```python
from build123d import *

# Parameters (mm, degrees)
F1_DEPTH  = 1066.8
F3_W      = 101.6
F3_H      = 50.8
F4_DEPTH  = 152.4
F5_W      = 101.6
F5_H      = 50.8
F6_DEPTH  = 177.801
F8_DEPTH  = 177.801
F10_W     = 101.6
F10_H     = 101.6
F11_DEPTH = 177.801


with BuildPart() as f1:
    # F0 (on Top) → F1 (new body)
    with BuildSketch(Plane.XY):
        Polygon((76.2, 0), (0, 0), (0, -152.4), (558.8, -152.4), (558.8, 0), (482.6, 0), (482.6, 25.4), (330.2, 25.4), (330.2, 0), (228.6, 0), (228.6, 25.4), (76.2, 25.4), align=None)
    extrude(amount=F1_DEPTH)

    # F3 (on offset) → F4 (join)
    with BuildSketch(Plane.XZ.offset(152.4)):
        with Locations((279.4, 1092.2)):
            Rectangle(F3_W, F3_H)
    extrude(amount=-F4_DEPTH)

    # F5 (on offset) → F6 (cut, through all)
    with BuildSketch(Plane.XZ.offset(152.4)):
        with Locations((279.4, 25.4)):
            Rectangle(F5_W, F5_H)
    extrude(amount=-F6_DEPTH, mode=Mode.SUBTRACT)

    # F7 (on offset) → F8 (cut, through all)
    with BuildSketch(Plane.XZ.offset(152.4)):
        Polygon((586.1058764434, 586.1058764434), (0, 0), (586.1058764434, 0), align=None)
    extrude(amount=-F8_DEPTH, mode=Mode.SUBTRACT)

    # F9: F1 across face


with BuildPart() as f1_1:
    add(f1.part)
    add(f1.part.mirror(Plane(origin=(279.4, -68.7916666667, 279.4), x_dir=(0, 1, 0), z_dir=(0.7071067812, 0, -0.7071067812))))

    # F10 (on offset) → F11 (cut, through all)
    with BuildSketch(Plane.XZ.offset(152.4)):
        with Locations((279.4, 1066.8)):
            Rectangle(F10_W, F10_H)
    extrude(amount=-F11_DEPTH, mode=Mode.SUBTRACT)


solid = f1_1.part
```
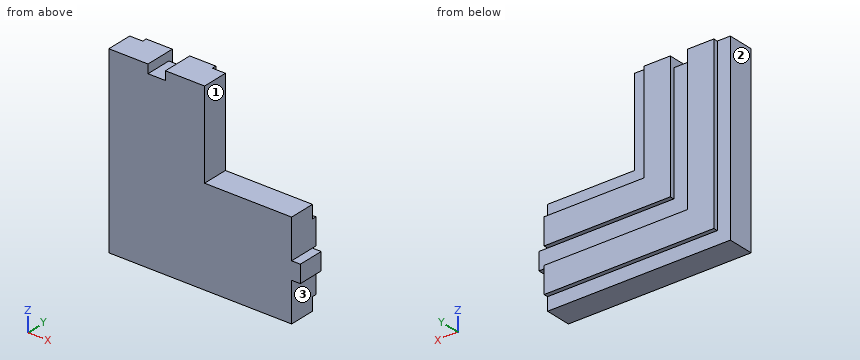
Input: part model. Units: mm. Frame: model coordinates. Face numbers are marked on the shaded views. A direction names the side the tool comes from. Round coordinates to 2 decimals unless told otherwise and drop trailing zeros. Loops run counter-clockwise (first coordinate to the right, second up) from the corner with the lowest first, then second, coordinate; pieces in that order, holes last. Notation, with made-up numbers: (-2.5, 21) -> (38.5, 21) arc R10 cw to (38.5, 39) -> close; hole circle Ø10 at (77.5, 33). An arc over 180 degrees is marked (long way). One line per item, written item: value.
(1) Material intervals for line 1 (Z direction, x = 677, y = 9); line 2 (X direction, y = -142.5, z = 534); line 3 (Z direction, x = 957, y = -5), sorted ascending. Write a range as [from, to].
Geometry check:
line 1: [76.2, 228.6], [330.2, 482.6]
line 2: [0, 1066.8]
line 3: [0, 558.8]
(2) Pin query (flat end, axial travel): pin 1 (7.5 mm diameter, centred on y = 6.5, z = 644, fed in from -X); pin 2 (5 mm diameter, centred on x = 294.5, y = -53.5, fed in from +Z); pin 3 (7.5 mm diameter, centred on x = 822.5, y = 17.5, fed in from +Z). Return the tip coordinate at first contact, or that it passes through.
Geometry check:
pin 1: x = 76.2
pin 2: z = 1016
pin 3: z = 482.6
(3) Section C-C (y = -99.5). Return the cut outline in (x, z).
Geometry check:
outline: (0, 0) -> (1066.8, 0) -> (1066.8, 228.6) -> (1117.6, 228.6) -> (1117.6, 330.2) -> (1066.8, 330.2) -> (1066.8, 558.8) -> (558.8, 558.8) -> (558.8, 1066.8) -> (330.2, 1066.8) -> (330.2, 1016) -> (228.6, 1016) -> (228.6, 1066.8) -> (0, 1066.8) -> close
(4) Set-up query: the marked faces 1, 2 and 3. Return all of +Z, -Z, +X, -X, +Y, -Y with unobstructed straight access to the full face (end or side cutting, diameter ignored); none if empty.
Geometry check:
face 1: +Z, +X, +Y, -Y
face 2: +Z, -Z, -X, +Y, -Y
face 3: -Z, +X, +Y, -Y
(5) Section B-B (x = 863). Return the cut outline in (y, z), plus the area to 3 significant figures.
Geometry check:
outline: (-152.4, 0) -> (0, 0) -> (0, 76.2) -> (25.4, 76.2) -> (25.4, 228.6) -> (0, 228.6) -> (0, 330.2) -> (25.4, 330.2) -> (25.4, 482.6) -> (0, 482.6) -> (0, 558.8) -> (-152.4, 558.8) -> close
area: 92,900 mm2
(6) Section A-A (z = 574). Return the cut outline in (x, y).
Geometry check:
outline: (0, -152.4) -> (558.8, -152.4) -> (558.8, 0) -> (482.6, 0) -> (482.6, 25.4) -> (330.2, 25.4) -> (330.2, 0) -> (228.6, 0) -> (228.6, 25.4) -> (76.2, 25.4) -> (76.2, 0) -> (0, 0) -> close
(7) Section D-D (z = 152.5). Return the cut outline in (x, y).
Geometry check:
outline: (0, -152.4) -> (1066.8, -152.4) -> (1066.8, 25.4) -> (76.2, 25.4) -> (76.2, 0) -> (0, 0) -> close
